The model under review builds one solid part; all positions refer to its coordinate system, in mm. A direction names the side the tool comes from. Give positions to 0.01 mm unless a question says otherwise; leave off trailing zeros. Order: outer loops, then holes, each group sorted by start corner. A loop starts at its lowest first (then second) coordinate and runs counter-clockwise, first axis right, second up. Notation, with made-up numbers: (56.5, 4.25) - (115.5, 4.25) arc R7 cw to (115.5, 9.25) - close; hole circle Ø6 at (-9.75, 60.25). An arc over 180 degrees is marked (long way). Answer as CSV lines item,"result". Start each with the question number.
from build123d import *

# Parameters (mm, degrees)
BOSS_EXTRUDE1_DEPTH = 5
SKETCH2_R           = 5
BOSS_EXTRUDE2_DEPTH = 11
BOSS_EXTRUDE3_DEPTH = 8
CUT_EXTRUDE1_DEPTH  = 42
SKETCH6_R           = 1.5
CUT_EXTRUDE2_DEPTH  = 32
LPATTERN1_COUNT     = 3
LPATTERN1_PITCH     = 7
FILLET1_R           = 0.5
FILLET2_R           = 5
FILLET3_R           = 0.5


with BuildPart() as part:
    # Sketch1 → Boss-Extrude1 (new body)
    with BuildSketch(Plane.XY):
        with BuildLine():
            ThreePointArc((10, 0), (0, 10), (-10, 0))
            ThreePointArc((-10, 0), (0, -10), (10, 0))
        make_face()
    extrude(amount=BOSS_EXTRUDE1_DEPTH)

    # Sketch2 → Boss-Extrude2 (add)
    with BuildSketch(Plane.XY):
        with Locations(Location((0, 0, 0), (0, 0, 180))):
            Circle(SKETCH2_R)
    extrude(amount=BOSS_EXTRUDE2_DEPTH)

    # Sketch3 → Boss-Extrude3 (add)
    with BuildSketch(Plane.XY.offset(11)):
        Polygon((10, -10), (30, -10), (30, 10), (10, 10), (-10, 10), (-10, -10), align=None)
    extrude(amount=BOSS_EXTRUDE3_DEPTH)

    # Sketch5 → Cut-Extrude1 (cut)
    with BuildSketch(Plane(origin=(-10, 0, 0), x_dir=(0, 0, -1), z_dir=(1, 0, 0))):
        Polygon((-19, 3), (-16, 6), (-16, -6), (-19, -3), align=None)
    extrude(amount=CUT_EXTRUDE1_DEPTH, mode=Mode.SUBTRACT)

    # Sketch6 → Cut-Extrude2 (cut)
    with BuildSketch(Plane.XY):
        with Locations((26.5, 0)):
            Circle(SKETCH6_R)
    cut_extrude2 = extrude(amount=CUT_EXTRUDE2_DEPTH, mode=Mode.SUBTRACT)

    # LPattern1: Cut-Extrude2 ×3
    with Locations(*[(-i * LPATTERN1_PITCH, 0, 0) for i in range(1, LPATTERN1_COUNT)]):
        add(cut_extrude2, mode=Mode.SUBTRACT)

    # Fillet1
    fillet1_edges = [part.edges().sort_by_distance(p)[0] for p in [
        (10, 3, 19),
        (10, -3, 19),
        (10, -6, 16),
        (10, 6, 16),
    ]]
    fillet(fillet1_edges, radius=FILLET1_R)

    # Fillet2
    # the kernel refuses this fillet: 5 mm, written as the material it takes off along each edge
    with BuildSketch(Plane(origin=(-10, -10, -1.5), x_dir=(1, 0, 0), z_dir=(0, 0, 1)), Plane(origin=(30, -10, -1.5), x_dir=(0, 1, 0), z_dir=(0, 0, 1))) as fillet2_piece_1:
        with BuildLine():
            CenterArc((FILLET2_R, FILLET2_R), FILLET2_R, 180, 90)
            Line((0, FILLET2_R), (0, 0))
            Line((0, 0), (FILLET2_R, 0))
        make_face()
    extrude(amount=33, mode=Mode.SUBTRACT)
    with BuildSketch(Plane(origin=(30, 10, -1.5), x_dir=(0, -1, 0), z_dir=(0, 0, 1)), Plane(origin=(-10, 10, -1.5), x_dir=(1, 0, 0), z_dir=(0, 0, 1))) as fillet2_piece_2:
        with BuildLine():
            CenterArc((FILLET2_R, -FILLET2_R), FILLET2_R, 90, 90)
            Line((0, -FILLET2_R), (0, 0))
            Line((0, 0), (FILLET2_R, 0))
        make_face()
    extrude(amount=33, mode=Mode.SUBTRACT)

    # Fillet3
    fillet3_edges = [part.edges().sort_by_distance(p)[0] for p in [
        (5, 0, 11),
        (10, 0, 0),
        (10, 0, 5),
        (5, 0, 5),
    ]]
    fillet(fillet3_edges, radius=FILLET3_R)


solid = part.part
Item 1: Machinability: for faces 4 (the face through (10, -5, 17)), 5 (the face through (4, -4, 5)), 6 (the face through (10, -7, 19)), which of the approach directions +Z, -Z, +X, -X, +Y, -Y give a long, thin tool a straight path to every point of the face, cutting with its end or side? Answer none if there is none.
Item 2: Clearance check with flat-ended pins moving along their axes: pin 1 (5 mm diameter, centred on x = 19.5, y = 0, fed in from -Z); pin 2 (4 mm diameter, centred on x = -1.5, y = -2, fed in from +Z); pin 3 (1.5 mm diameter, centred on y = 1.5, z = 9.5, fed in from +X). State where each tip first meets the part, or that it passes through.
Item 3: Take a section at C-C on x = 0. Write out the cut boundary in (y, z).
Item 4: Take a section at A-A on x = 19.5. Write out the cut boundary in (y, z).
Item 5: Mouldability with a two-part tool opening along Z and no side actions: class faces 1 (the face through (0, 0, 0)), 2 (the face through (10.28, 3.75, 18.7)), 3 (the face through (-10, 0, 13)) as released by +Z, released by -Z, zero draft, split by the parting line, or undercut.
Item 6: For line 1 along X through (y, z) = (0, 12.6); line 2 along Y through (x, z) = (12.5, 14.4); line 3 along Z through (x, y) = (1, 6.25), list the stretches that pass through material, from the lowest coordinate up.
Item 7: Take a section at B-B on z = 15.25. Write out the cut boundary in (x, y), and give its area (3 significant figures).
Item 8: Take a section at D-D on x = 26.5. Write out the cut boundary in (y, z).
Data:
1,face 4,"+X, -X"
1,face 5,"none"
1,face 6,"+Z, +X, -X, +Y, -Y"
2,pin 1,"stops at z = 11"
2,pin 2,"stops at z = 18.96"
2,pin 3,"stops at x = 4.94"
3,outline,"(-10, 0.5) arc R0.5 ccw to (-9.5, 0) - (9.5, 0) arc R0.5 ccw to (10, 0.5) - (10, 4.5) arc R0.5 ccw to (9.5, 5) - (5.5, 5) arc R0.5 cw to (5, 5.5) - (5, 10.5) arc R0.5 cw to (5.5, 11) - (10, 11) - (10, 19) - (4.21, 19) arc R0.5 ccw to (3.85, 18.15) - (5.15, 16.85) arc R0.5 cw to (4.79, 16) - (-4.79, 16) arc R0.5 cw to (-5.15, 16.85) - (-3.85, 18.15) arc R0.5 ccw to (-4.21, 19) - (-10, 19) - (-10, 11) - (-5.5, 11) arc R0.5 cw to (-5, 10.5) - (-5, 5.5) arc R0.5 cw to (-5.5, 5) - (-9.5, 5) arc R0.5 ccw to (-10, 4.5) - close"
4,outline,"(-10, 11) - (-1.5, 11) - (-1.5, 16) - (-4.79, 16) arc R0.5 cw to (-5.15, 16.85) - (-3.85, 18.15) arc R0.5 ccw to (-4.21, 19) - (-10, 19) - close; (1.5, 11) - (10, 11) - (10, 19) - (4.21, 19) arc R0.5 ccw to (3.85, 18.15) - (5.15, 16.85) arc R0.5 cw to (4.79, 16) - (1.5, 16) - close"
5,face 1,"released by -Z"
5,face 2,"undercut"
5,face 3,"zero draft"
6,line 1,"x = -10 to 11, 14 to 18, 21 to 25, 28 to 30"
6,line 2,"y = -10 to -1.5, 1.5 to 10"
6,line 3,"z = 0 to 5, 11 to 19"
7,outline,"(-10, -5) arc R5 ccw to (-5, -10) - (25, -10) arc R5 ccw to (30, -5) - (30, 5) arc R5 ccw to (25, 10) - (-5, 10) arc R5 ccw to (-10, 5) - close; hole circle Ø3 at (12.5, 0); hole circle Ø3 at (19.5, 0); hole circle Ø3 at (26.5, 0)"
7,area,"757 mm^2"
8,outline,"(-9.77, 11) - (-1.5, 11) - (-1.5, 16) - (-4.79, 16) arc R0.5 cw to (-5.15, 16.85) - (-3.85, 18.15) arc R0.5 ccw to (-4.21, 19) - (-9.77, 19) - close; (1.5, 11) - (9.77, 11) - (9.77, 19) - (4.21, 19) arc R0.5 ccw to (3.85, 18.15) - (5.15, 16.85) arc R0.5 cw to (4.79, 16) - (1.5, 16) - close"
